CAD build for the part. Positions are in the model's coordinates, mm. Face numbers are marked on the shaded views. A direction names the side the tool comes from. Give positions to 0.01 mm unless a question says otherwise; leave off trailing zeros. Loops run counter-clockwise (first coordinate to the right, second up) from the corner with the lowest first, then second, coordinate; pieces in that order, holes last.
Item 1: Saw through at B-B on y = -4.75. Give the cut face in (x, z).
Item 2: Which spindle directions (+Z, -Z, +X, -X, +Y, -Y) get a long thin tool onto all of the face, cutting with end or side? Do the marked faces 5 and 6. Say none if no direction does.
Item 3: Drop flat-ended pins along their axis: P1, Ø2, axis at x = 18.5, z = 10.5, coming from the +Y side; P2, Ø12, axis at x = 13.5, z = 37, coming from the -Y side; P3, Ø7.5, axis at y = -2.3, z = 15, coming from the -X side; P4, Ø5, axis at x = -9.5, y = -3, coming from the -Z side. Give the stop position or say it passes through.
Item 4: Probe probe 1 along X at (y, z) = (-6.25, 11.5); probe 2 along Z at (x, y) = (-15, 0.25); probe 3 along Y at (x, z) = (16.5, 9.5). List the from-to ranges inside material, lowest first.
Item 5: Mould opens along X. For the marked faces 1, 2, 3 and 4 say: released by +X, released by -X, zero draft, split by the parting line, or undercut.
Item 6: Saw through at D-D on z = 41.5. Give the cut face in (x, y).
Item 7: Saw through at A-A on z = 15. Give the cut face in (x, y).
Item 8: Saw through at C-C on z = 23. Give the cut face in (x, y), plus the area to 3 significant figures.
from build123d import *

# Parameters (mm, degrees)
BOSS_EXTRUDE1_DEPTH = 60
SKETCH2_R           = 4.25
CUT_EXTRUDE1_DEPTH  = 9.704955679


with BuildPart() as part:
    # Sketch1 → Boss-Extrude1 (new body)
    with BuildSketch(Plane.XY):
        with BuildLine():
            Line((-23.304685018, 17.700444455), (-23.304685018, -12.299555545))
            Line((-23.304685018, -12.299555545), (-13.599729339, -12.299555545))
            Line((-13.599729339, -12.299555545), (-13.599729339, 4.700444455))
            Line((-13.599729339, 4.700444455), (26.990359303, 4.700444455))
            Line((26.990359303, 4.700444455), (26.990359303, -12.299555545))
            Line((26.990359303, -12.299555545), (36.695314982, -12.299555545))
            Line((36.695314982, -12.299555545), (36.695314982, 17.700444455))
            Line((36.695314982, 17.700444455), (25.501661634, 17.700444455))
            Line((25.501661634, 17.700444455), (26.990359303, 15.121944455))
            ThreePointArc((26.990359303, 15.121944455), (26.990359303, 14.740944455), (26.660403624, 14.550444455))
            Line((26.660403624, 14.550444455), (-13.26977366, 14.550444455))
            ThreePointArc((-13.26977366, 14.550444455), (-13.599729339, 14.740944455), (-13.599729339, 15.121944455))
            Line((-13.599729339, 15.121944455), (-12.11103167, 17.700444455))
            Line((-12.11103167, 17.700444455), (-23.304685018, 17.700444455))
        make_face()
    extrude(amount=BOSS_EXTRUDE1_DEPTH)

    # Sketch2 → Cut-Extrude1 (cut)
    with BuildSketch(Plane.ZY.offset(23.304685018)):
        with Locations(Location((15, -2.299555545, 0), (0, 0, 270))):
            Circle(SKETCH2_R)
        with Locations(Location((45, -2.299555545, 0), (0, 0, 270))):
            Circle(SKETCH2_R)
    extrude(amount=-CUT_EXTRUDE1_DEPTH, mode=Mode.SUBTRACT)


solid = part.part
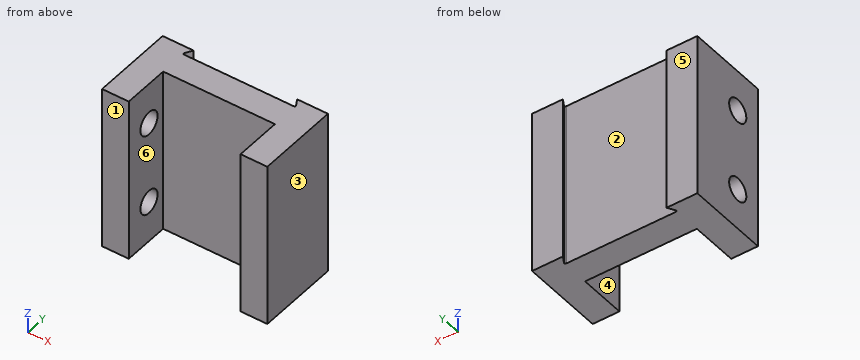
Results below:
1. outline: (-23.3, 0) - (-13.6, 0) - (-13.6, 11.53) - (-23.3, 11.53) - close; (-23.3, 18.47) - (-13.6, 18.47) - (-13.6, 41.53) - (-23.3, 41.53) - close; (-23.3, 48.47) - (-13.6, 48.47) - (-13.6, 60) - (-23.3, 60) - close; (26.99, 0) - (36.7, 0) - (36.7, 60) - (26.99, 60) - close
2. face 5: +Z, -Z, +X, -X, +Y
2. face 6: +Z, -Z, -Y
3. P1: stops at y = 14.55
3. P2: stops at y = 4.7
3. P3: stops at x = 26.99
3. P4: passes through
4. probe 1: x = -23.3 to -13.6, 26.99 to 36.7
4. probe 2: z = 0 to 11.6, 18.4 to 41.6, 48.4 to 60
4. probe 3: y = 4.7 to 14.55
5. face 1: zero draft
5. face 2: undercut
5. face 3: released by +X
5. face 4: undercut
6. outline: (-23.3, -12.3) - (-13.6, -12.3) - (-13.6, -4.71) - (-23.3, -4.71) - close; (-23.3, 0.11) - (-13.6, 0.11) - (-13.6, 4.7) - (26.99, 4.7) - (26.99, -12.3) - (36.7, -12.3) - (36.7, 17.7) - (25.5, 17.7) - (26.99, 15.12) arc R0.38 cw to (26.66, 14.55) - (-13.27, 14.55) arc R0.38 cw to (-13.6, 15.12) - (-12.11, 17.7) - (-23.3, 17.7) - close
7. outline: (-23.3, -12.3) - (-13.6, -12.3) - (-13.6, -6.55) - (-23.3, -6.55) - close; (-23.3, 1.95) - (-13.6, 1.95) - (-13.6, 4.7) - (26.99, 4.7) - (26.99, -12.3) - (36.7, -12.3) - (36.7, 17.7) - (25.5, 17.7) - (26.99, 15.12) arc R0.38 cw to (26.66, 14.55) - (-13.27, 14.55) arc R0.38 cw to (-13.6, 15.12) - (-12.11, 17.7) - (-23.3, 17.7) - close
8. outline: (-23.3, -12.3) - (-13.6, -12.3) - (-13.6, 4.7) - (26.99, 4.7) - (26.99, -12.3) - (36.7, -12.3) - (36.7, 17.7) - (25.5, 17.7) - (26.99, 15.12) arc R0.38 cw to (26.66, 14.55) - (-13.27, 14.55) arc R0.38 cw to (-13.6, 15.12) - (-12.11, 17.7) - (-23.3, 17.7) - close
8. area: 986 mm2
